Autodesk Inventor part; units mm, degrees
ref_plane "YZ Plane" through (0, 0, 0) normal (1, 0, 0) x (0, 1, 0)
ref_plane "XZ Plane" through (0, 0, 0) normal (0, 1, 0) x (-1, 0, 0)
ref_plane "XY Plane" through (0, 0, 0) normal (0, 0, 1) x (1, 0, 0)
sketch "스케치1" plane through (0, 0, 0) normal (0, 0, 1) x (1, 0, 0)
  circle A0 centre (0, 0) radius 20
  dimension "d0" = 40
extrude "돌출1" add sketch "스케치1" along normal blind 7
sketch "스케치2" plane through (0, 0, 7) normal (0, 0, 1) x (1, 0, 0)
  circle A0 centre (0, 0) radius 20
  line L0 (17.3205, 10) -> (17.3205, -10)
  line L1 (17.3205, -10) -> (200, -10)
  line L2 (200, -10) -> (200, 10)
  line L3 (200, 10) -> (17.3205, 10)
  dimension "d4" = 10
  dimension "d5" = 20
  dimension "d8" = 200
extrude "돌출2" add sketch "스케치2" against normal blind 7 contours A0 L3 L2 L1
sketch "스케치3" plane through (0, 0, 7) normal (0, 0, 1) x (1, 0, 0)
  circle A0 centre (0, 0) radius 14
  circle A1 centre (14, 0) radius 1.55
  dimension "d9" = 28
  dimension "d10" = 3.1
hole "구멍1" at (14, 0, 7) direction (0, 0, -1) diameter 3.1 depth 20 countersink diameter 6.5 countersink angle 90
pattern_circular "원형 패턴1" count 6 over 360 about axis through (0, 0, 0) along (0, 0, 1) of "구멍1"
fillet "모깎기1" radius 6 2 edges at (17.3205, 10, 3.5) (17.3205, -10, 3.5)
sketch "스케치4" plane through (0, 0, 7) normal (0, 0, 1) x (1, 0, 0)
  line L0 (20.4939, -10) -> (200, -10)
  line L1 (20.4939, 10) -> (200, 10)
  line L2 (200, -10) -> (192, -10)
  line L3 (192, -10) -> (192, 10)
  line L4 (192, 10) -> (200, 10)
  line L5 (200, 10) -> (200, -10)
  line L6 (196, 10) -> (196, -10)
  circle A0 centre (196, 5) radius 1.5
  circle A1 centre (196, -5) radius 1.5
  point P0 (0, 0)
  dimension "d22" = 8
  dimension "d23" = 3
  dimension "d24" = 3
  dimension "d25" = 5
  dimension "d26" = 10
  dimension "d27" = 5
hole "구멍2" at (196, 5, 7) at (196, -5, 7) direction (0, 0, -1) diameter 3.1 depth 20 countersink diameter 6.5 countersink angle 90
properties part number "test_arm_2"
Geometry: final body of the model. Coordinates: model frame, mm. A direction names the side the tool comes from. Round coordinates to 2 decimals unless told otherwise and drop trailing zeros. Write each loop counter-clockwise with the first axis right and the second up, starting at its lowest first coordinate (ties: lowest second). Pieces come first, ordered by that corner, then holes. Notation, with made-up numbers: (26.25, -22) -> (66.25, -22) arc R13 ccw to (66.25, -15) -> close; hole circle Ø7 at (-23.5, -13). An arc over 180 degrees is marked (long way). Use CSV: the item, a comma, the result in double quotes. Start each with the question number.
Q1. Section B-B (x = 92). Return loops of the section in (y, z), plus the area to 3 significant figures.
Q2. First-contact query: pin 1 Ø5 at (x, y) = (196, -5) entering from +Z; pin 2 Ø4 at (x, y) = (-14, 0) entering from +Z; pin 3 Ø3.5 at (x, z) = (145, 3) entering from -Y. Flat tips, straight axial feed; report the tip coordinate or a pass-through.
Q3. Section A-A (z = 1.5). Give the number of separate pieces and of enclosed holes in the cut face, plus the area to 3 significant figures.
Q4. Line query: L1, parallel to X at y = 1.5, z = 6; L2, parallel to Y at x = 5.5, z = 6.25; L3, parallel to Y at x = 14, z = 3.35. Output: solid intervals per line, ascending.
Q5. Pull-direction query (X, two-part tool) for faces 3 (the face through (5.88, -13.35, 5.41)), 4 (the face through (109, -10, 4)), 5 (the face through (-19.99, -0.69, 3.45)), 6 (the face through (194.38, -4.64, 5.41)); classes: pulls with the +X half, pulls with the -X half, needs draft (parallel to the pull), parting line crosses it, or undercut.
Q6. Reachability of faces 1 (the face through (112, 10, 4)), 2 (the face through (194.38, 5.36, 5.41)) from +Z, -Z, +X, -X, +Y, -Y: full face, straight path, thin tool, end or side. Return the list, or none.
Result sheet:
1,outline,"(-10, 0) -> (10, 0) -> (10, 7) -> (-10, 7) -> close"
1,area,"140 mm²"
2,pin 1,"z = 6.25"
2,pin 2,"z = 5.75"
2,pin 3,"y = -10"
3,separate pieces,"1"
3,enclosed holes,"8"
3,area,"4,820 mm²"
4,L1,"-19.94 to -15.68, -12.32 to 12.32, 15.68 to 200"
4,L2,"-19.23 to -14.12, -10.12 to 10.12, 14.12 to 19.23"
4,L3,"-14.28 to -1.55, 1.55 to 14.28"
5,face 3,"undercut"
5,face 4,"needs draft"
5,face 5,"parting line crosses it"
5,face 6,"undercut"
6,face 1,"+Z, -Z, +X, +Y"
6,face 2,"+Z"
